Autodesk Inventor part; units mm, degrees
ref_plane "to_bolt_row_1_to_3_XY" through (1, 21, 5) normal (0, 0, 1) x (1, 0, 0)
ref_plane "to_bolt_row_1_to_3_YZ" through (1, 21, 5) normal (1, 0, 0) x (0, 1, 0)
ref_plane "to_bolt_row_1_to_3_ZX" through (1, 21, 5) normal (0, 1, 0) x (0, 0, 1)
sketch "Sketch_15" plane through (0, 0, 0) normal (1, 0, 0) x (0, 1, 0)
  line L0 (0, 28) -> (0, 0)
  line L1 (0, 0) -> (28, 0)
  line L2 (28, 0) -> (28, 4.5858)
  arc A0 (28, 4.5858) -> (27.7071, 5.2929) centre (27, 4.5858) ccw
  line L3 (27.7071, 5.2929) -> (5.2929, 27.7071)
  arc A1 (5.2929, 27.7071) -> (4.5858, 28) centre (4.5858, 27) ccw
  line L4 (4.5858, 28) -> (0, 28)
extrude "Extrusion1" add sketch "Sketch_15" along normal mid plane 12
sketch "Sketch_60" plane through (0, -1, 0) normal (0, 1, 0) x (1, 0, 0)
  line L0 (-6, 0) -> (-6, -28)
  line L1 (-6, -28) -> (6, -28)
  line L2 (6, -28) -> (6, 0)
  line L3 (6, 0) -> (-6, 0)
extrude "Extrusion2" add sketch "Sketch_60" along normal blind 1
sketch "Sketch_61" plane through (0, -1, 0) normal (0, 1, 0) x (1, 0, 0)
  line L0 (-6, 0) -> (-6, -28)
  line L1 (-6, -28) -> (6, -28)
  line L2 (6, -28) -> (6, 0)
  line L3 (6, 0) -> (-6, 0)
  arc A0 (-2, -10.7) -> (-1.7, -11) centre (-1.7, -10.7) ccw
  line L4 (-1.7, -11) -> (3.7, -11)
  arc A1 (3.7, -11) -> (4, -10.7) centre (3.7, -10.7) ccw
  line L5 (4, -10.7) -> (4, -5.3)
  arc A2 (4, -5.3) -> (3.7, -5) centre (3.7, -5.3) ccw
  line L6 (3.7, -5) -> (-1.7, -5)
  arc A3 (-1.7, -5) -> (-2, -5.3) centre (-1.7, -5.3) ccw
  line L7 (-2, -5.3) -> (-2, -10.7)
  arc A4 (-2, -24.7) -> (-1.7, -25) centre (-1.7, -24.7) ccw
  line L8 (-1.7, -25) -> (3.7, -25)
  arc A5 (3.7, -25) -> (4, -24.7) centre (3.7, -24.7) ccw
  line L9 (4, -24.7) -> (4, -22.3)
  arc A6 (4, -22.3) -> (3.7, -22) centre (3.7, -22.3) ccw
  line L10 (3.7, -22) -> (-1.7, -22)
  arc A7 (-1.7, -22) -> (-2, -22.3) centre (-1.7, -22.3) ccw
  line L11 (-2, -22.3) -> (-2, -24.7)
extrude "Extrusion3" cut sketch "Sketch_61" along normal blind 1
sketch "Sketch_62" plane through (0, 0, 0) normal (0, 0, 1) x (1, 0, 0)
  line L0 (-6, 0) -> (6, 0)
  line L1 (6, 0) -> (6, 28)
  line L2 (6, 28) -> (-6, 28)
  line L3 (-6, 28) -> (-6, 0)
extrude "Extrusion4" add sketch "Sketch_62" along normal mid plane 2
sketch "Sketch_63" plane through (0, 0, -1) normal (0, 0, 1) x (1, 0, 0)
  line L0 (-6, 0) -> (6, 0)
  line L1 (6, 0) -> (6, 28)
  line L2 (6, 28) -> (-6, 28)
  line L3 (-6, 28) -> (-6, 0)
  line L4 (-2, 10.7) -> (-2, 5.3)
  arc A0 (-2, 5.3) -> (-1.7, 5) centre (-1.7, 5.3) ccw
  line L5 (-1.7, 5) -> (3.7, 5)
  arc A1 (3.7, 5) -> (4, 5.3) centre (3.7, 5.3) ccw
  line L6 (4, 5.3) -> (4, 10.7)
  arc A2 (4, 10.7) -> (3.7, 11) centre (3.7, 10.7) ccw
  line L7 (3.7, 11) -> (-1.7, 11)
  arc A3 (-1.7, 11) -> (-2, 10.7) centre (-1.7, 10.7) ccw
  line L8 (-2, 24.7) -> (-2, 22.3)
  arc A4 (-2, 22.3) -> (-1.7, 22) centre (-1.7, 22.3) ccw
  line L9 (-1.7, 22) -> (3.7, 22)
  arc A5 (3.7, 22) -> (4, 22.3) centre (3.7, 22.3) ccw
  line L10 (4, 22.3) -> (4, 24.7)
  arc A6 (4, 24.7) -> (3.7, 25) centre (3.7, 24.7) ccw
  line L11 (3.7, 25) -> (-1.7, 25)
  arc A7 (-1.7, 25) -> (-2, 24.7) centre (-1.7, 24.7) ccw
extrude "Extrusion5" cut sketch "Sketch_63" along normal blind 1
sketch "Sketch_12" plane through (-4, 0, 0) normal (1, 0, 0) x (0, 0, -1)
  line L0 (-28, 5) -> (-16.5, 5)
  arc A0 (-16.5, 5) -> (-16, 5.5) centre (-16.5, 5.5) ccw
  line L1 (-16, 5.5) -> (-16, 14)
  arc A1 (-14, 16) -> (-16, 14) centre (-14, 14) ccw
  line L2 (-14, 16) -> (-5.5, 16)
  arc A2 (-5.5, 16) -> (-5, 16.5) centre (-5.5, 16.5) ccw
  line L3 (-5, 16.5) -> (-5, 28)
  line L4 (-5, 28) -> (-28, 28)
  line L5 (-28, 28) -> (-28, 5)
extrude "Extrusion6" cut sketch "Sketch_12" along normal blind 16
sketch "Sketch_20" plane through (0, 0, 0) normal (0, 0, 1) x (1, 0, 0)
  circle A0 centre (1, 21) radius 2.6
extrude "Extrusion7" cut sketch "Sketch_20" along normal mid plane 10
sketch "Sketch_29" plane through (0, 0, 0) normal (0, 1, 0) x (-1, 0, 0)
  circle A0 centre (-1, 21) radius 2.6
extrude "Extrusion8" cut sketch "Sketch_29" along normal mid plane 10
ref_plane "to_bolt_row_1_to_3_XY" through (1, 21, 5) normal (0, 0, 1) x (1, 0, 0)
ref_plane "to_bolt_row_1_to_3_YZ" through (1, 21, 5) normal (1, 0, 0) x (0, 1, 0)
ref_plane "to_bolt_row_1_to_3_ZX" through (1, 21, 5) normal (0, 1, 0) x (0, 0, 1)
ref_plane "to_bolt_row_1_to_3_base_XY" through (1, 5, 21) normal (0, 1, 0) x (1, 0, 0)
ref_plane "to_bolt_row_1_to_3_base_YZ" through (1, 5, 21) normal (1, 0, 0) x (0, 0, -1)
ref_plane "to_bolt_row_1_to_3_base_ZX" through (1, 5, 21) normal (0, 0, -1) x (0, 1, 0)
ref_plane "to_nut_row_1_to_3_XY" through (1, 21, -2) normal (0, 0, 1) x (1, 0, 0)
ref_plane "to_nut_row_1_to_3_YZ" through (1, 21, -2) normal (1, 0, 0) x (0, 1, 0)
ref_plane "to_nut_row_1_to_3_ZX" through (1, 21, -2) normal (0, 1, 0) x (0, 0, 1)
ref_plane "to_nut_row_1_to_3_base_XY" through (1, -2, 21) normal (0, 1, 0) x (1, 0, 0)
ref_plane "to_nut_row_1_to_3_base_YZ" through (1, -2, 21) normal (1, 0, 0) x (0, 0, -1)
ref_plane "to_nut_row_1_to_3_base_ZX" through (1, -2, 21) normal (0, 0, -1) x (0, 1, 0)
ref_plane "bracket_to_dummy_XY" through (0, 0, 0) normal (0, 1, 0) x (1, 0, 0)
ref_plane "bracket_to_dummy_YZ" through (0, 0, 0) normal (1, 0, 0) x (0, 0, -1)
ref_plane "bracket_to_dummy_ZX" through (0, 0, 0) normal (0, 0, -1) x (0, 1, 0)
ref_plane "bracket_to_bolt_XY" through (1, 21, 0) normal (0, 0, 1) x (1, 0, 0)
ref_plane "bracket_to_bolt_YZ" through (1, 21, 0) normal (1, 0, 0) x (0, 1, 0)
ref_plane "bracket_to_bolt_ZX" through (1, 21, 0) normal (0, 1, 0) x (0, 0, 1)
properties part number "HBLFSL5hblfsn5"
Build history of the part. All positions in model axes, mm. A direction names the side the tool comes from. Round coordinates to 2 decimals unless told otherwise and drop trailing zeros. Order: outer loops, then holes, each group sorted by start corner. A loop starts at its lowest first (then second) coordinate and runs counter-clockwise, first axis right, second up. Notation, with made-up numbers: (-25, 44.5) -> (22, 44.5) arc R19 cw to (22, 66.5) -> close; hole circle Ø8 at (-36, 44). An arc over 180 degrees is marked (long way). Answer in a Markdown table with one row per item.
1) Band-saw the part on B-B on y = 21. Give the cut face in (x, z).
Values:
| item | result |
|---|---|
| outline | (-6, 0) -> (-1.6, 0) -> (-1.6, 5) -> (-4, 5) -> (-4, 12) -> (-6, 12) -> close; (3.6, 0) -> (6, 0) -> (6, 5) -> (3.6, 5) -> close |
2) Band-saw the part on A-A on x = 1. Give the number of separate pieces and of enclosed holes in the cut face, and give its area (3 significant figures).
Values:
| item | result |
|---|---|
| separate pieces | 3 |
| enclosed holes | 0 |
| area | 338 mm2 |
3) Mould opens along X. For faces 1 (the cylindrical face through (0.44, 23.54, 2.62)), 2 (the flat face through (4, 8, -0.5)), 3 (the flat face through (1, -1, 8)) say: released by +X, released by -X, zero draft, split by the parting line, or undercut.
Values:
| item | result |
|---|---|
| face 1 | undercut |
| face 2 | released by +X |
| face 3 | zero draft |
4) Pin check, flat tips, straight feed: P1, Ø0.5, axis at y = 8, z = -0.5, coming from the +X side; P2, Ø0.8, axis at y = -0.5, z = 9.5, coming from the -X side; P3, Ø3, axis at x = -1, z = 22, coming from the +Y side; P4, Ø1.1, axis at x = 0, y = -0.5, coming from the +Z side. Stop position of each tip, or through.
Values:
| item | result |
|---|---|
| P1 | x = 4 |
| P2 | x = -2 |
| P3 | y = 5 |
| P4 | z = 28 |
5) Band-saw the part on C-C on y = 7.75. Give the cut face in (x, z).
Values:
| item | result |
|---|---|
| outline | (-6, 0) -> (-2, 0) -> (-2, -1) -> (4, -1) -> (4, 0) -> (6, 0) -> (6, 16) -> (-4, 16) -> (-4, 25.25) -> (-6, 25.25) -> close |
6) Which spindle directions (+Z, -Z, +X, -X, +Y, -Y) get a long thin tool onto all of the face, cutting with end or side? Do faces 4 (the flat face through (1, -0.5, 11)), 5 (the flat face through (-2, 23.5, -0.5)), 6 (the flat face through (1, 5, -0.5)), 7 (the flat face through (1, 25, 5)). Say none if no direction does.
Values:
| item | result |
|---|---|
| face 4 | +X, -X, -Y |
| face 5 | -Z, -X, +Y, -Y |
| face 6 | -Z, +X, -X, -Y |
| face 7 | +Z, +X, +Y |
7) Wall check: L1, parallel to X at y = 21, z = 2.15; L2, parallel to Z at x = 1, y = 2.15; L3, parallel to Z at x = -2.25, y = 0.75. Give the ranges that are in metal, low to high.
Values:
| item | result |
|---|---|
| L1 | -6 to -1.6, 3.6 to 6 |
| L2 | 0 to 18.4, 23.6 to 28 |
| L3 | 0 to 28 |
8) Band-saw the part on D-D on z = 24. Give the cut face in (x, y).
Values:
| item | result |
|---|---|
| outline | (-6, 0) -> (-2, 0) -> (-2, -1) -> (4, -1) -> (4, 0) -> (6, 0) -> (6, 5) -> (-4, 5) -> (-4, 9) -> (-6, 9) -> close |
